Build history of the part. All positions in model axes, mm. Round coordinates to 2 decimals unless told otherwise and drop trailing zeros. Order: outer loops, then holes, each group sorted by start corner. A loop starts at its lowest first (then second) coordinate and runs counter-clockwise, first axis right, second up. Notation, with made-up numbers: (-17.5, 57.25) -> (-8.5, 57.25) arc R16 cw to (-8.5, 86.25) -> close; hole circle Ø2 at (34, 0). An arc over 180 degrees is marked (long way). Answer as a JSON object with one key per item and string values.
Autodesk Inventor part; units mm, degrees
ref_plane "YZ Plane" through (0, 0, 0) normal (1, 0, 0) x (0, 1, 0)
ref_plane "XZ Plane" through (0, 0, 0) normal (0, 1, 0) x (-1, 0, 0)
ref_plane "XY Plane" through (0, 0, 0) normal (0, 0, 1) x (1, 0, 0)
sketch "Sketch1" plane through (0, 0, 0) normal (0, 1, 0) x (-1, 0, 0)
  circle A0 centre (0, 0) radius 10
  dimension "d0" = 20
extrude "Extrusion1" add sketch "Sketch1" along normal blind 1050
sketch "Sketch2" plane through (0, 0, 0) normal (0, -1, 0) x (1, 0, 0)
  circle A0 centre (0, 0) radius 10
  circle A1 centre (0, 0) radius 17.5
  dimension "d3" = 35
extrude "Extrusion2" add sketch "Sketch2" along normal blind 25 contours A0 | A1
sketch "Sketch3" plane through (0, -25, 0) normal (0, -1, 0) x (1, 0, 0)
  circle A0 centre (0, 0) radius 22.5
  dimension "d6" = 45
extrude "Extrusion3" add sketch "Sketch3" along normal blind 5
sketch "Sketch4" plane through (0, 1050, 0) normal (0, 1, 0) x (1, 0, 0)
  circle A0 centre (0, 0) radius 12.5
  dimension "d9" = 25
extrude "Extrusion4" add sketch "Sketch4" along normal blind 15
properties part number "linear_rod"
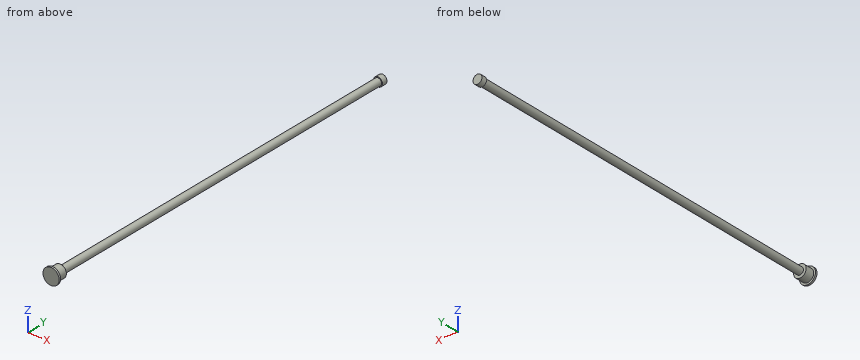
1) Cut at A-A, the plane z = 0. Give the cut face in (x, y).
Checked values:
{"outline": "(-22.5, -30) -> (22.5, -30) -> (22.5, -25) -> (17.5, -25) -> (17.5, 0) -> (10, 0) -> (10, 1050) -> (12.5, 1050) -> (12.5, 1065) -> (-12.5, 1065) -> (-12.5, 1050) -> (-10, 1050) -> (-10, 0) -> (-17.5, 0) -> (-17.5, -25) -> (-22.5, -25) -> close"}
2) Cut at C-C, the plane y = 952. Give the cut face in (x, z), plus the area to 3 significant figures.
Checked values:
{"outline": "circle Ø20 at (0, 0)", "area": "314 mm²"}
3) Probe L1, parallel to Y at x = 8.5, z = -8.5; L2, parallel to Y at x = 17, z = 11.5; L3, parallel to Y at x = -12.5, z = 10.5. List the from-to ranges inside material, lowest first. Write a range as from..to.
Checked values:
{"L1": "y = -30..0, 1050..1065", "L2": "y = -30..-25", "L3": "y = -30..0"}
4) Flat gauge pins, fed straight in: pin 1 Ø1 at (y, z) = (605, -9.5) entering from -X; pin 2 Ø5 at (y, z) = (794.5, 3.5) entering from +X; pin 3 Ø5 at (y, z) = (365, 0) entering from +X; pin 4 Ø8 at (x, y) = (-15, 258) entering from +Z. Where does each tip first touch, or does it go through?
Checked values:
{"pin 1": "stops at x = -4.36", "pin 2": "stops at x = 9.95", "pin 3": "stops at x = 10", "pin 4": "passes through"}
5) Cut at B-B, the plane x = 0. Give the cut face in (y, z), plus the area to 3 significant figures.
Checked values:
{"outline": "(-30, -22.5) -> (-25, -22.5) -> (-25, -17.5) -> (0, -17.5) -> (0, -10) -> (1050, -10) -> (1050, -12.5) -> (1065, -12.5) -> (1065, 12.5) -> (1050, 12.5) -> (1050, 10) -> (0, 10) -> (0, 17.5) -> (-25, 17.5) -> (-25, 22.5) -> (-30, 22.5) -> close", "area": "22,500 mm²"}
